Part model, mm, in its own coordinate system. Round coordinates to 2 decimals unless told otherwise and drop trailing zeros. Write each loop counter-clockwise with the first axis right and the second up, starting at its lowest first coordinate (ties: lowest second). Pieces come first, ordered by that corner, then holes. Notation, with made-up numbers: M -15.5,60.5 L -5.5,60.5 A9 cw -5.5,75.5 Z; hole C 56.5,-0.75 d9. An arc over 180 degrees is marked long. Use one line per item in the form item = value. Start each with the question number.
Item 1: Probe L1, parallel to X at y = -17, z = -33; L2, parallel to X at y = -4.25, z = -25.5; L3, parallel to X at y = -7.5, z = -15.5. List the from-to ranges inside material, lowest first.
Item 2: Flat gauge pin, fed straight in: pin 1 Ø1 at (x, y) = (-32.5, -18) entering from -Z. Where does the tip first touch, or does it go through?
Item 3: Cut at B-B, the plane y = -12.75. Give the cut face in (x, z).
Item 4: Cut at C-C, the plane y = -5.5. State how many separate pieces and enclosed holes the cut face has, then the cut area to 3 significant figures.
Item 5: Cut at A-A, the plane z = -2. Give the cut face in (x, y), then the cut area to 3 significant figures.
from build123d import *

# Parameters (mm, degrees)
F0_W     = 95
F0_H     = 95
F1_DEPTH = 8
F2_R     = 1.55
F3_DEPTH = 8.001
F5_DEPTH = 8.001
F6_R     = 5
F7_DEPTH = 20
F8_R     = 1.5
F9_DEPTH = 20.001
F11_R    = 5
F12_R    = 1


with BuildPart() as f1:
    # F0 (on Front) → F1 (new body)
    with BuildSketch(Plane.XZ):
        Rectangle(F0_W, F0_H)
    extrude(amount=F1_DEPTH)

    # F2 (on face) → F3 (cut, through all)
    with BuildSketch(Plane.XZ.offset(8)):
        with Locations((-43.2573593129, 43.2573593129)):
            Circle(F2_R)
        with Locations((-43.2573593129, -43.2573593129)):
            Circle(F2_R)
        with Locations((43.2573593129, -43.2573593129)):
            Circle(F2_R)
        with Locations((43.2573593129, 43.2573593129)):
            Circle(F2_R)
    extrude(amount=-F3_DEPTH, mode=Mode.SUBTRACT)

    # F4 (on face) → F5 (cut, through all)
    with BuildSketch(Plane.XZ.offset(8)):
        Polygon((-44.5, 19.1396103068), (-44.5, 0), (-44.5, -19.1396103068), (-31.8198051534, -31.8198051534), (-19.1396103068, -44.5), (0, -44.5), (19.1396103068, -44.5), (31.8198051534, -31.8198051534), (44.5, -19.1396103068), (44.5, 0), (44.5, 19.1396103068), (31.8198051534, 31.8198051534), (19.1396103068, 44.5), (0, 44.5), (-19.1396103068, 44.5), (-31.8198051534, 31.8198051534), align=None)
        with BuildLine():
            ThreePointArc((-39.4552751314, 44.5), (-39.2609809541, 43.0871828943), (-39.5746770207, 41.6959973642))
            Line((-39.5746770207, 41.6959973642), (-32.8804653252, 35.0017856687))
            Line((-32.8804653252, 35.0017856687), (-23.3822509939, 44.5))
            Line((-23.3822509939, 44.5), (-39.4552751314, 44.5))
        make_face()
        with BuildLine():
            Line((-44.5, 23.3822509939), (-35.0017856687, 32.8804653252))
            Line((-35.0017856687, 32.8804653252), (-41.6959973642, 39.5746770207))
            ThreePointArc((-41.6959973642, 39.5746770207), (-43.0871828943, 39.2609809541), (-44.5, 39.4552751314))
            Line((-44.5, 39.4552751314), (-44.5, 23.3822509939))
        make_face()
        with BuildLine():
            Line((-32.8804653252, -35.0017856687), (-39.5746770207, -41.6959973642))
            ThreePointArc((-39.5746770207, -41.6959973642), (-39.2609809541, -43.0871828943), (-39.4552751314, -44.5))
            Line((-39.4552751314, -44.5), (-23.3822509939, -44.5))
            Line((-23.3822509939, -44.5), (-32.8804653252, -35.0017856687))
        make_face()
        with BuildLine():
            ThreePointArc((-44.5, -39.4552751314), (-43.0871828943, -39.2609809541), (-41.6959973642, -39.5746770207))
            Line((-41.6959973642, -39.5746770207), (-35.0017856687, -32.8804653252))
            Line((-35.0017856687, -32.8804653252), (-44.5, -23.3822509939))
            Line((-44.5, -23.3822509939), (-44.5, -39.4552751314))
        make_face()
        with BuildLine():
            Line((35.0017856687, -32.8804653252), (41.6959973642, -39.5746770207))
            ThreePointArc((41.6959973642, -39.5746770207), (43.0871828943, -39.2609809541), (44.5, -39.4552751314))
            Line((44.5, -39.4552751314), (44.5, -23.3822509939))
            Line((44.5, -23.3822509939), (35.0017856687, -32.8804653252))
        make_face()
        with BuildLine():
            ThreePointArc((39.4552751314, -44.5), (39.2609809541, -43.0871828943), (39.5746770207, -41.6959973642))
            Line((39.5746770207, -41.6959973642), (32.8804653252, -35.0017856687))
            Line((32.8804653252, -35.0017856687), (23.3822509939, -44.5))
            Line((23.3822509939, -44.5), (39.4552751314, -44.5))
        make_face()
        with BuildLine():
            Line((32.8804653252, 35.0017856687), (39.5746770207, 41.6959973642))
            ThreePointArc((39.5746770207, 41.6959973642), (39.2609809541, 43.0871828943), (39.4552751314, 44.5))
            Line((39.4552751314, 44.5), (23.3822509939, 44.5))
            Line((23.3822509939, 44.5), (32.8804653252, 35.0017856687))
        make_face()
        with BuildLine():
            ThreePointArc((44.5, 39.4552751314), (43.0871828943, 39.2609809541), (41.6959973642, 39.5746770207))
            Line((41.6959973642, 39.5746770207), (35.0017856687, 32.8804653252))
            Line((35.0017856687, 32.8804653252), (44.5, 23.3822509939))
            Line((44.5, 23.3822509939), (44.5, 39.4552751314))
        make_face()
    extrude(amount=-F5_DEPTH, mode=Mode.SUBTRACT)

    # F6 (on face) → F7 (join)
    with BuildSketch(Plane(origin=(0, 0, 0), x_dir=(-1, 0, 0), z_dir=(0, 1, 0))):
        with Locations((-32.8804653252, 32.8804653252)):
            Circle(F6_R)
        with Locations((-32.8804653252, -32.8804653252)):
            Circle(F6_R)
        with Locations((32.8804653252, -32.8804653252)):
            Circle(F6_R)
        with Locations((32.8804653252, 32.8804653252)):
            Circle(F6_R)
    extrude(amount=-F7_DEPTH)

    # F8 (on face) → F9 (cut, through all)
    with BuildSketch(Plane.XZ.offset(20)):
        with Locations((-32.8804653252, -32.8804653252)):
            Circle(F8_R)
        with Locations((32.8804653252, -32.8804653252)):
            Circle(F8_R)
        with Locations((32.8804653252, 32.8804653252)):
            Circle(F8_R)
        with Locations((-32.8804653252, 32.8804653252)):
            Circle(F8_R)
    extrude(amount=-F9_DEPTH, mode=Mode.SUBTRACT)

    # F11
    f11_edges = [f1.edges().sort_by_distance(p)[0] for p in [
        (-47.5, -4, 47.5),
        (47.5, -4, 47.5),
        (47.5, -4, -47.5),
        (-47.5, -4, -47.5),
    ]]
    fillet(f11_edges, radius=F11_R)

    # F12
    f12_edges = [f1.edges().sort_by_distance(p)[0] for p in [
        (-39.455275, -4, 44.5),
        (-39.574677, -4, 41.695997),
        (-23.382251, -4, 44.5),
        (-30.568441, -4, 37.31381),
        (-35.19249, -4, 37.31381),
        (-37.31381, -4, 35.19249),
        (-37.31381, -4, 30.568441),
        (-44.5, -4, 23.382251),
        (-41.695997, -4, 39.574677),
        (-44.5, -4, 39.455275),
        (-44.5, -4, 19.13961),
        (-19.13961, -4, 44.5),
        (-28.447121, -4, 35.19249),
        (-35.19249, -4, 28.447121),
        (30.568441, -4, 37.31381),
        (35.19249, -4, 37.31381),
        (44.5, -4, 23.382251),
        (19.13961, -4, 44.5),
        (35.19249, -4, 28.447121),
        (28.447121, -4, 35.19249),
        (44.5, -4, 19.13961),
        (39.455275, -4, 44.5),
        (41.695997, -4, 39.574677),
        (44.5, -4, 39.455275),
        (37.31381, -4, 30.568441),
        (23.382251, -4, 44.5),
        (39.574677, -4, 41.695997),
        (37.31381, -4, 35.19249),
        (44.5, -4, -19.13961),
        (28.447121, -4, -35.19249),
        (35.19249, -4, -28.447121),
        (19.13961, -4, -44.5),
        (37.31381, -4, -30.568441),
        (37.31381, -4, -35.19249),
        (44.5, -4, -23.382251),
        (35.19249, -4, -37.31381),
        (30.568441, -4, -37.31381),
        (44.5, -4, -39.455275),
        (41.695997, -4, -39.574677),
        (39.574677, -4, -41.695997),
        (39.455275, -4, -44.5),
        (23.382251, -4, -44.5),
        (-19.13961, -4, -44.5),
        (-28.447121, -4, -35.19249),
        (-35.19249, -4, -28.447121),
        (-44.5, -4, -19.13961),
        (-23.382251, -4, -44.5),
        (-30.568441, -4, -37.31381),
        (-39.455275, -4, -44.5),
        (-39.574677, -4, -41.695997),
        (-35.19249, -4, -37.31381),
        (-37.31381, -4, -35.19249),
        (-37.31381, -4, -30.568441),
        (-44.5, -4, -23.382251),
        (-41.695997, -4, -39.574677),
        (-44.5, -4, -39.455275),
    ]]
    fillet(f12_edges, radius=F12_R)


solid = f1.part
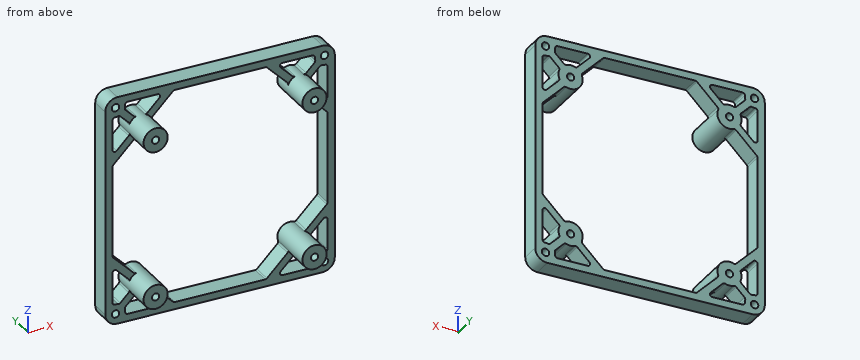
Model answer:
q1.L1 = -37.88 to -34.38, -31.39 to -27.88, 27.88 to 31.39, 34.38 to 37.88
q1.L2 = -47.5 to -44.46, -42.38 to -38.14, 38.14 to 42.38, 44.46 to 47.5
q1.L3 = -47.5 to -44.5, 44.5 to 47.5
q2.pin_1 = -37.88
q3.outline = C -32.88,-32.88 d10; C -32.88,32.88 d10; C 32.88,-32.88 d10; C 32.88,32.88 d10; hole C -32.88,-32.88 d3; hole C -32.88,32.88 d3; hole C 32.88,-32.88 d3; hole C 32.88,32.88 d3
q4.separate_pieces = 1
q4.enclosed_holes = 17
q4.area = 1,790 mm²
q5.outline = M -47.5,-8 L -44.5,-8 L -44.5,0 L -47.5,0 Z; M 44.5,-8 L 47.5,-8 L 47.5,0 L 44.5,0 Z
q5.area = 48.0 mm²
